```python
from build123d import *

# Parameters (mm, degrees)
SKETCH1_R               = 30
BOSS_EXTRUDE1_DEPTH     = 5
SKETCH2_R               = 19.5
BOSS_EXTRUDE2_DEPTH     = 1
SKETCH3_R               = 17.5
BOSS_EXTRUDE3_DEPTH     = 15
SKETCH4_R               = 12.025
CUT_EXTRUDE1_DEPTH      = 7
SKETCH5_R               = 10.5
CUT_EXTRUDE2_DEPTH      = 45.676615807
CUT_EXTRUDE3_DEPTH      = 4
CUT_EXTRUDE3_DEPTH_BACK = 4
CUT_EXTRUDE3_START      = -5
SKETCH6_R               = 2
SKETCH7_R               = 1.75
CUT_EXTRUDE4_DEPTH      = 10
SKETCH8_R               = 1.225
CUT_EXTRUDE5_DEPTH      = 12


with BuildPart() as part:
    # Sketch1 → Boss-Extrude1 (new body)
    with BuildSketch(Plane.XY):
        Circle(SKETCH1_R)
    extrude(amount=BOSS_EXTRUDE1_DEPTH)

    # Sketch2 → Boss-Extrude2 (add)
    with BuildSketch(Plane.XY.offset(5)):
        Circle(SKETCH2_R)
    extrude(amount=BOSS_EXTRUDE2_DEPTH)

    # Sketch3 → Boss-Extrude3 (add)
    with BuildSketch(Plane.XY.offset(6)):
        Circle(SKETCH3_R)
    extrude(amount=BOSS_EXTRUDE3_DEPTH)

    # Sketch4 → Cut-Extrude1 (cut)
    with BuildSketch(Plane(origin=(0, 0, 0), x_dir=(-1, 0, 0), z_dir=(0, 0, -1))):
        Circle(SKETCH4_R)
    extrude(amount=-CUT_EXTRUDE1_DEPTH, mode=Mode.SUBTRACT)

    # Sketch5 → Cut-Extrude2 (cut, through all)
    with BuildSketch(Plane(origin=(0, 0, 7), x_dir=(-1, 0, 0), z_dir=(0, 0, -1))):
        Circle(SKETCH5_R)
    extrude(amount=-CUT_EXTRUDE2_DEPTH, mode=Mode.SUBTRACT)

    # Sketch6 → Cut-Extrude3 (cut, two sides: drawn at the far end of the back side and taken through both)
    with BuildSketch(Plane.XY.offset(5).offset(CUT_EXTRUDE3_START - CUT_EXTRUDE3_DEPTH_BACK)):
        with Locations((24.5, 0)):
            Circle(SKETCH6_R)
        with Locations((12.25, -21.217622393)):
            Circle(SKETCH6_R)
        with Locations((-12.25, -21.217622393)):
            Circle(SKETCH6_R)
        with Locations((-24.5, 0)):
            Circle(SKETCH6_R)
        with Locations((-12.25, 21.217622393)):
            Circle(SKETCH6_R)
        with Locations((12.25, 21.217622393)):
            Circle(SKETCH6_R)
    extrude(amount=CUT_EXTRUDE3_DEPTH + CUT_EXTRUDE3_DEPTH_BACK, mode=Mode.SUBTRACT)

    # Sketch7 → Cut-Extrude4 (cut)
    with BuildSketch(Plane.XY.offset(21)):
        with Locations((14, 0)):
            Circle(SKETCH7_R)
        with Locations((7, -12.124355653)):
            Circle(SKETCH7_R)
        with Locations((-7, -12.124355653)):
            Circle(SKETCH7_R)
        with Locations((-14, 0)):
            Circle(SKETCH7_R)
        with Locations((-7, 12.124355653)):
            Circle(SKETCH7_R)
        with Locations((7, 12.124355653)):
            Circle(SKETCH7_R)
    extrude(amount=-CUT_EXTRUDE4_DEPTH, mode=Mode.SUBTRACT)

    # Sketch8 → Cut-Extrude5 (cut)
    with BuildSketch(Plane.XY.offset(21)):
        with Locations((12.124355653, 7)):
            Circle(SKETCH8_R)
        with Locations((0, -14)):
            Circle(SKETCH8_R)
        with Locations((-12.124355653, 7)):
            Circle(SKETCH8_R)
    extrude(amount=-CUT_EXTRUDE5_DEPTH, mode=Mode.SUBTRACT)


solid = part.part
```
Geometry: final body of the model. Coordinates: model frame, mm. A direction names the side the tool comes from. Round coordinates to 2 decimals unless told otherwise and drop trailing zeros. Order: outer loops, then holes, each group sorted by start corner. A loop starts at its lowest first (then second) coordinate and runs counter-clockwise, first axis right, second up. Notation, with made-up numbers: M 6.5,67.5 L 13.5,67.5 A24 ccw 13.5,100.5 Z; hole C 56.25,62 d7. An arc over 180 degrees is marked long. One line per item, written item: value.
(1) Cut plane B-B (y = 9). Return the cut outline in (x, z) (3 decimals).
Result sheet:
outline: M -28.618,0 L -7.975,0 L -7.975,7 L -5.408,7 L -5.408,21 L -15.008,21 L -15.008,6 L -17.299,6 L -17.299,5 L -28.618,5 Z; M 5.408,7 L 7.975,7 L 7.975,0 L 28.618,0 L 28.618,5 L 17.299,5 L 17.299,6 L 15.008,6 L 15.008,21 L 5.408,21 Z
(2) Line query: probe 1 along Y at (x, z) = (0, 11.75) (3 decimals); probe 2 along Y at (x, z) = (12.25, 1.2); probe 3 along X at (y, z) = (0.5, 18). Output: solid intervals per line, ascending. Write a range as [from, to].
Result sheet:
probe 1: [-17.5, -15.225], [-12.775, -10.5], [10.5, 17.5]
probe 2: [-27.38, -23.22], [-19.22, 19.22], [23.22, 27.38]
probe 3: [-17.49, -15.68], [-12.32, -10.49], [10.49, 12.32], [15.68, 17.49]
(3) Reachability of faces 1 (the cylindrical face through (-5.38, -12.79, 16.07)), 2 (the flat face through (24, 0, 4)), 3 (the cylindrical face through (-10, 3.2, 13.9)) from +Z, -Z, +X, -X, +Y, -Y: full face, straight path, thin tool, end or side. Return the list, or none.
Result sheet:
face 1: +Z
face 2: -Z
face 3: +Z, -Z
(4) Cut plane A-A (x = 0). Return the cut outline in (y, z) (3 decimals).
Result sheet:
outline: M -30,0 L -12.025,0 L -12.025,7 L -10.5,7 L -10.5,21 L -12.775,21 L -12.775,9 L -15.225,9 L -15.225,21 L -17.5,21 L -17.5,6 L -19.5,6 L -19.5,5 L -30,5 Z; M 10.5,7 L 12.025,7 L 12.025,0 L 30,0 L 30,5 L 19.5,5 L 19.5,6 L 17.5,6 L 17.5,21 L 10.5,21 Z
(5) Pin query (flat end, axial travel): P1, Ø1, axis at x = 7, y = -11.5, coming from the +Z side; P2, Ø3, axis at y = -4.5, z = 17, coming from the +X side; P3, Ø10, axis at x = 13.5, z = 10.5, coming from the +Y side. Return the tip coordinate at first contact, or that it passes through.
Result sheet:
P1: z = 11
P2: x = 17.24
P3: y = 15.88
(6) Cut plane C-C (x = -24.5). Return the cut outline in (y, z).
Result sheet:
outline: M -17.31,0 L -2,0 L -2,4 L 2,4 L 2,0 L 17.31,0 L 17.31,5 L -17.31,5 Z
(7) Cut plane D-D (y = -22). Return the cut outline in (x, z), and give its area (3 significant figures).
Result sheet:
outline: M -20.4,0 L -14.09,0 L -14.09,4 L -10.41,4 L -10.41,0 L 10.41,0 L 10.41,4 L 14.09,4 L 14.09,0 L 20.4,0 L 20.4,5 L -20.4,5 Z
area: 175 mm2
(8) Pull-direction query (X, two-part tool) for faces 4 (the cylindrical face through (-29.97, 1.32, 2.46)), 5 (the flat face through (-14, 0, 11)), 6 (the flat face through (0, -20, 5)); classes: pulls with the +X half, pulls with the -X half, needs draft (parallel to the pull), parting line crosses it, or undercut.
Result sheet:
face 4: parting line crosses it
face 5: undercut
face 6: needs draft
